Geometry: final body of the model. Coordinates: model frame, mm. A direction names the side the tool comes from. Round coordinates to 2 decimals unless told otherwise and drop trailing zeros. Loops run counter-clockwise (first coordinate to the right, second up) from the corner with the lowest first, then second, coordinate; pieces in that order, holes last. Notation, with made-up numbers: M -33,54 L -21,54 A17 ccw -21,75 Z; hole C 84,-30.75 d7. An arc over 180 degrees is marked long. Return JSON: item names as keys, results as strings.
Autodesk Fusion 360 part; units mm, degrees
sketch "Sketch1" plane through (0, 0, 0) normal (0, 1, 0) x (1, 0, 0)
  line L0 (0, 0) -> (27.5, 0)
  line L1 (27.5, 0) -> (27.5, -30)
  line L2 (27.5, -30) -> (19.5, -30)
  line L3 (19.5, -30) -> (19.5, -20)
  line L4 (19.5, -20) -> (7.5, -20)
  line L5 (7.5, -20) -> (7.5, -5)
  line L6 (7.5, -5) -> (0, -5)
  line L7 (0, -5) -> (0, 0)
  line L8 (19, -30) -> (19, -28)
  line L9 (19, -28) -> (7, -28)
  line L10 (7, -28) -> (7, -12)
  line L11 (7, -12) -> (0, -12)
  line L12 (0, -12) -> (0, -30)
  line L13 (0, -30) -> (19, -30)
  line L14 (27.5, -30) -> (18.2223, -30)
  line L15 (27.5, -35) -> (27.5, -30)
  line L16 (15.5, -35) -> (15.5, -32)
  line L17 (11, -30) -> (27.5, -30)
  line L18 (15.5, -35) -> (27.5, -35)
  line L19 (19.5, -30) -> (19.5, -32)
  line L20 (19.5, -32) -> (15.5, -32)
  dimension "d1" = 7.5
  dimension "d2" = 27.5
  dimension "d3" = 30
  dimension "d4" = 8
  dimension "d5" = 10
  dimension "d6" = 5
  dimension "d8" = 19
  dimension "d9" = 2
  dimension "d10" = 18
  dimension "d11" = 7
  dimension "d13" = 12
  dimension "d15" = 3
  dimension "d16" = 2
  dimension "d21" = 11
revolve "Revolve1" add sketch "Sketch1" angle 360 about axis through (0, 0, 1.75) along (0, 0, 1) contours L0 L1 L2 L3 L4 L5 L6 L7 L14 L17 makes body 1
revolve "Revolve2" add sketch "Sketch1" angle 360 about axis through (0, 0, 5) along (0, 0, -1) separate body contours L2 L14 L15 L16 L17 L18 L19 L20 makes body 2
revolve "Revolve3" add sketch "Sketch1" angle 360 about axis through (0, 0, 12) along (0, 0, 1) separate body contours L8 L9 L10 L11 L12 L13 L14 L17 makes body 3
chamfer "Chamfer1" distance 2 angle 45 1 edges at (-6.5263, -2.5313, 12) on bodies 3
chamfer "Chamfer2" distance 1 angle 45 1 edges at (-25.639, -9.9444, 35) on bodies 2
sketch "Sketch2" plane through (0, 0, 35) normal (0, 0, 1) x (-1, 0, 0)
  circle A0 centre (0, 0) radius 15.5
  circle A1 centre (0, 0) radius 26.5
  circle A2 centre (0, 0) radius 23.5 construction
  circle A3 centre (0, 0) radius 27.5
  line L0 (0, 0) -> (-19, 0)
  line L1 (0, 0) -> (0, -32) construction
  circle A4 centre (0, -23.5) radius 1
  circle A5 centre (20.3516, 11.75) radius 1
  circle A6 centre (-20.3516, 11.75) radius 1
  dimension "d22" = 2
  dimension "d24" = 360
  dimension "d30" = 50
  dimension "d31" = 32
  dimension "d32" = 47
hole "Hole1" at (-20.3516, -11.75, 35) at (0, 23.5, 35) at (20.3516, -11.75, 35) direction (0, 0, -1) diameter 2 depth 16 tip angle 118 countersink diameter 6 countersink angle 90 bodies 1 2 3
hole "Hole2" at (27.5, 0, 29.9966) direction (-1, 0, 0) diameter 2 depth 10 tip angle 118 bodies 1 2
component "Body" placed x (1, 0, 0) y (0, 1, 0) z (0, 0, 1) at (0, 0, 0)
component "Retaininer" placed x (1, 0, 0) y (0, 1, 0) z (0, 0, 1) at (0, 0, 0)
component "Plunger" placed x (1, 0, 0) y (0, 1, 0) z (0, 0, 1) at (0, 0, 0)
hidden bodies 2 3
equation "d1 = ( 15 / 2 ) * 1 mm"
equation "d2 = ( 55 / 2 ) * 1 mm"
equation "d8 = d2 - d4 - 0.5 mm"
equation "d10 = d3 - d5 - 2 mm"
equation "d11 = d1 - 0.5 mm"
equation "d13 = d4 + 4 mm"
equation "d32 = 55 mm - 8 mm"
Q1. Section query D-D (y = 0). Output: boundary loops of the cut face in (x, z), plus the area to 3 significant figures.
Determined:
{"outline": "M -27.5,0 L 27.5,0 L 27.5,29 L 19.5,29 L 19.5,20 L 7.5,20 L 7.5,5 L -7.5,5 L -7.5,20 L -19.5,20 L -19.5,30 L -27.5,30 Z", "area": "1,030 mm^2"}
Q2. Pin query (flat end, axial travel): pin 1 (8 mm diameter, centred on x = 1, z = 9.5, fed in from -Y); pin 2 (6 mm diameter, centred on y = -15, z = 7, fed in from +X); pin 3 (1.2 mm diameter, centred on x = -20.35, y = -11.75, fed in from +Z). Return the tip coordinate at first contact, or that it passes through.
Determined:
{"pin 1": "stops at y = -27.5", "pin 2": "stops at x = 24.74", "pin 3": "stops at z = 18.76"}
Q3. Reachability of faces 1 (the cylindrical face through (18.6, -5.86, 24.93)), 2 (the flat face through (0, 0, 0)) from +Z, -Z, +X, -X, +Y, -Y: full face, straight path, thin tool, end or side. Return the list, or none.
Determined:
{"face 1": "+Z", "face 2": "-Z, +X, -X, +Y, -Y"}
Q4. Section query C-C (x = -13.5). Output: boundary loops of the cut face in (y, z).
Determined:
{"outline": "M -23.96,0 L 23.96,0 L 23.96,30 L 14.07,30 L 14.07,20 L -14.07,20 L -14.07,30 L -23.96,30 Z"}
Q5. Section query B-B (y = -16). Output: boundary loops of the cut face in (x, z), plus the area to 3 significant figures.
Determined:
{"outline": "M -22.37,0 L 22.37,0 L 22.37,30 L 11.15,30 L 11.15,20 L -11.15,20 L -11.15,30 L -22.37,30 Z", "area": "1,120 mm^2"}
Q6. Material intervals for L1, parallel to Y at x = 0, z = 26.25; L2, parallel to Y at x = 0, z = 10; L3, parallel to X at y = -11.75, z = 28, sorted ascending.
Determined:
{"L1": "y = -27.5 to -19.5, 19.5 to 22.5, 24.5 to 27.5", "L2": "y = -27.5 to -7.5, 7.5 to 27.5", "L3": "x = -24.86 to -21.35, -19.35 to -15.56, 15.56 to 19.35, 21.35 to 24.86"}
Q7. Section query A-A (z = 6.5). Output: boundary loops of the cut face in (x, y).
Determined:
{"outline": "C 0,0 d55; hole C 0,0 d15"}
